```python
from build123d import *

# Parameters (mm, degrees)
BOSS_EXTRUDE1_DEPTH = 2
SKETCH1_3_W         = 42.3
SKETCH1_3_H         = 2
BOSS_EXTRUDE2_DEPTH = 25.4
SKETCH1_4_W         = 8.8
SKETCH1_4_H         = 4
BOSS_EXTRUDE3_DEPTH = 25.3
FILLET31_R          = 3
FILLET32_R          = 2.36
FILLET26_R          = 2.2
SKETCH2_R           = 2
CUT_EXTRUDE1_DEPTH  = 10
SKETCH3_R           = 1.5
CUT_EXTRUDE2_DEPTH  = 10
SKETCH4_R           = 1.5
CUT_EXTRUDE3_DEPTH  = 10


with BuildPart() as part:
    # Sketch1 → Boss-Extrude1 (new body)
    with BuildSketch(Plane.XY):
        with BuildLine():
            Line((21.15, 16.48), (-21.15, 16.48))
            Line((-21.15, 16.48), (-21.15, 9.72))
            Line((-21.15, 9.72), (-29.95, 9.72))
            Line((-29.95, 9.72), (-29.95, -10.78))
            Line((-29.95, -10.78), (-21.15, -10.78))
            Line((-21.15, -10.78), (-21.15, -14.78))
            Line((-21.15, -14.78), (-18.337899039, -14.78))
            ThreePointArc((-18.337899039, -14.78), (-16.826007676, -17.431106014), (-13.96, -18.48))
            Line((-13.96, -18.48), (13.96, -18.48))
            ThreePointArc((13.96, -18.48), (16.826007676, -17.431106014), (18.337899039, -14.78))
            Line((18.337899039, -14.78), (21.15, -14.78))
            Line((21.15, -14.78), (21.15, -10.78))
            Line((21.15, -10.78), (29.95, -10.78))
            Line((29.95, -10.78), (29.95, 9.72))
            Line((29.95, 9.72), (21.15, 9.72))
            Line((21.15, 9.72), (21.15, 16.48))
        make_face()
    extrude(amount=BOSS_EXTRUDE1_DEPTH)

    # Sketch1_3 → Boss-Extrude2 (add)
    with BuildSketch(Plane.XY):
        with Locations((0, 17.48)):
            Rectangle(SKETCH1_3_W, SKETCH1_3_H)
    extrude(amount=BOSS_EXTRUDE2_DEPTH)

    # Sketch1_4 → Boss-Extrude3 (add)
    with BuildSketch(Plane.XY):
        with Locations((-25.55, -12.78)):
            Rectangle(SKETCH1_4_W, SKETCH1_4_H)
        with Locations((25.55, -12.78)):
            Rectangle(SKETCH1_4_W, SKETCH1_4_H)
    extrude(amount=BOSS_EXTRUDE3_DEPTH)

    # Fillet31
    fillet31_edges = [part.edges().sort_by_distance(p)[0] for p in [
        (21.15, -12.78, 2),
        (-29.95, 9.72, 1),
        (-21.15, 9.72, 1),
        (21.15, 9.72, 1),
        (29.95, 9.72, 1),
        (21.15, 17.48, 25.4),
        (-21.15, 17.48, 25.4),
        (-21.15, -12.78, 25.3),
        (-29.95, -12.78, 25.3),
        (-21.15, -12.78, 2),
        (29.95, -12.78, 25.3),
        (21.15, -12.78, 25.3),
    ]]
    fillet(fillet31_edges, radius=FILLET31_R)

    # Fillet32
    fillet32_edges = [part.edges().sort_by_distance(p)[0] for p in [
        (24.05, -10.78, 2),
        (0, 16.48, 2),
        (-24.05, -10.78, 2),
    ]]
    fillet(fillet32_edges, radius=FILLET32_R)

    # Fillet26
    fillet26_edges = [part.edges().sort_by_distance(p)[0] for p in [
        (0, 18.48, 0),
    ]]
    fillet(fillet26_edges, radius=FILLET26_R)

    # Sketch2 → Cut-Extrude1 (cut, symmetric)
    with BuildSketch(Plane.XZ.offset(14.78)):
        with Locations(Location((25.05, 19.14, 0), (0, 0, 270))):
            Circle(SKETCH2_R)
        with Locations(Location((25.05, 9.14, 0), (0, 0, 270))):
            Circle(SKETCH2_R)
        with Locations(Location((-25.15, 19.14, 0), (0, 0, 180))):
            Circle(SKETCH2_R)
        with Locations(Location((-25.15, 9.14, 0), (0, 0, 180))):
            Circle(SKETCH2_R)
    extrude(amount=CUT_EXTRUDE1_DEPTH, both=True, mode=Mode.SUBTRACT)

    # Sketch3 → Cut-Extrude2 (cut)
    with BuildSketch(Plane(origin=(0, 18.48, 0), x_dir=(1, 0, 0), z_dir=(0, 1, 0))):
        with Locations(Location((-9.134575671, -14.14, 0), (0, 0, 270))):
            Circle(SKETCH3_R)
        with Locations(Location((-9.134575671, -7.14, 0), (0, 0, 270))):
            Circle(SKETCH3_R)
        with Locations(Location((-2.134575671, -14.14, 0), (0, 0, 270))):
            Circle(SKETCH3_R)
        with Locations(Location((-9.134575671, -21.14, 0), (0, 0, 270))):
            Circle(SKETCH3_R)
        with Locations(Location((-16.134575671, -14.14, 0), (0, 0, 270))):
            Circle(SKETCH3_R)
        with Locations(Location((9.034575671, -14.14, 0), (0, 0, 270))):
            Circle(SKETCH3_R)
        with Locations(Location((9.034575671, -7.14, 0), (0, 0, 270))):
            Circle(SKETCH3_R)
        with Locations(Location((16.034575671, -14.14, 0), (0, 0, 270))):
            Circle(SKETCH3_R)
        with Locations(Location((9.034575671, -21.14, 0), (0, 0, 270))):
            Circle(SKETCH3_R)
        with Locations(Location((2.034575671, -14.14, 0), (0, 0, 270))):
            Circle(SKETCH3_R)
    extrude(amount=-CUT_EXTRUDE2_DEPTH, mode=Mode.SUBTRACT)

    # Sketch4 → Cut-Extrude3 (cut)
    with BuildSketch(Plane(origin=(0, 0, 0), x_dir=(-1, 0, 0), z_dir=(0, 0, -1))):
        with Locations((-7, -4.52)):
            Circle(SKETCH4_R)
        with Locations((0, 2.48)):
            Circle(SKETCH4_R)
        with Locations((7, -4.52)):
            Circle(SKETCH4_R)
        with Locations((0, -11.52)):
            Circle(SKETCH4_R)
        with Locations((0, -4.52)):
            Circle(SKETCH4_R)
    extrude(amount=-CUT_EXTRUDE3_DEPTH, mode=Mode.SUBTRACT)


solid = part.part
```
Verification items for the finished model (mm, model axes). A direction names the side the tool comes from. Give positions to 0.01 mm unless a question says otherwise; leave off trailing zeros. Loops run counter-clockwise (first coordinate to the right, second up) from the corner with the lowest first, then second, coordinate; pieces in that order, holes last. Notation, with made-up numbers: M 7,-33 L 24,-33 A7 cw 24,-23 Z; hole C -23,27 d7. An arc over 180 degrees is marked long. One line per question, with ' | ' between items.
Item 1: Tool access check on faces 1 (the face through (-21.15, 17, 9)), 2 (the face through (21.15, 17, 9)), 3 (the face through (25, -10.78, 15)), 4 (the face through (-26, -13, 25.3)), 5 (the face through (-9.07, 17.49, 12.64)). Record the directions out of +Z, -Z, +X, -X, +Y, -Y that give a thin tool (end or side, any length) a straight path to the whole face; none if there is none.
Completed:
face 1: +Z, -Z, -X, +Y | face 2: +Z, -Z, +X, +Y | face 3: +Z, +X, -X, +Y | face 4: +Z, +X, -X, +Y, -Y | face 5: +Y, -Y
Item 2: Section check D-D, the plane z = 3.5. Record the cut outline in (x, y), plus the area to 3 significant figures.
Completed:
outline: M -29.95,-14.78 L -20.75,-14.78 L -20.75,-10.62 L -29.95,-10.62 Z; M -21.15,16.32 L 21.15,16.32 L 21.15,18.48 L -21.15,18.48 Z; M 20.75,-14.78 L 29.95,-14.78 L 29.95,-10.62 L 20.75,-10.62 Z | area: 168 mm^2
Item 3: Section check C-C, the plane y = 2.48. Record the cut outline in (x, z).
Completed:
outline: M -29.95,0 L -1.5,0 L -1.5,2 L -29.95,2 Z; M 1.5,0 L 29.95,0 L 29.95,2 L 1.5,2 Z
Item 4: Draft check along Y on faces 6 (the face through (8.19, -5.43, 0.99)), 7 (the face through (7.704, 17.494, 7.832)), 8 (the face through (25, -14.78, 12)). Enter one of: +Y half, -Y half, draft (parallel to the pull), parting line (faces both ways), or undercut.
Completed:
face 6: undercut | face 7: draft | face 8: -Y half
Item 5: Thickness scan on line 1 (Z direction, x = -25.15, y = -12.3); line 2 (X direction, y = -13.45, z = 9.14); line 3 (Y direction, x = -7, z = 1.05). Record the ranges inside material, lowest first. Write a range as [from, to].
Completed:
line 1: z = [0, 7.14], [11.14, 17.14], [21.14, 25.3] | line 2: x = [-29.95, -27.15], [-23.15, -21.15], [21.15, 23.05], [27.05, 29.95] | line 3: y = [-18.48, -6.02], [-3.02, 18.16]
Item 6: Section check B-B, the plane x = -25.15. Record the cut outline in (y, z), plus the area to 3 significant figures.
Completed:
outline: M -14.78,0 L 9.72,0 L 9.72,2 L -8.42,2 A2.36 cw -10.78,4.36 L -10.78,7.14 L -14.78,7.14 Z; M -14.78,11.14 L -10.78,11.14 L -10.78,17.14 L -14.78,17.14 Z; M -14.78,21.14 L -10.78,21.14 L -10.78,25.3 L -14.78,25.3 Z | area: 111 mm^2
Item 7: Depth check by flat-ended pin: P1, Ø12, axis at x = -9, y = -7.5, coming from the +Z side; P2, Ø7, axis at x = -27, z = 16.5, coming from the +Y side; P3, Ø8, axis at x = 14, z = 16, coming from the -Y side; P4, Ø2.5, axis at x = -16.13, z = 14.14, coming from the -Y side. Enter the tip coordinate at first touch or a pass-through.
Completed:
P1: stops at z = 2 | P2: stops at y = -10.78 | P3: stops at y = 16.48 | P4: passes through
Item 8: Section check A-A, the plane y = -11.52. Record the cut outline in (x, z).
Completed:
outline: M -29.95,0 L -1.5,0 L -1.5,2 L -18.15,2 A3 cw -21.15,5 L -21.15,22.3 A3 ccw -24.15,25.3 L -26.95,25.3 A3 ccw -29.95,22.3 Z; M 1.5,0 L 29.95,0 L 29.95,22.3 A3 ccw 26.95,25.3 L 24.15,25.3 A3 ccw 21.15,22.3 L 21.15,5 A3 cw 18.15,2 L 1.5,2 Z; hole C -25.15,9.14 d4; hole C -25.15,19.14 d4; hole C 25.05,9.14 d4; hole C 25.05,19.14 d4
